Work out the finished part from the listing and answer in its coordinate system (mm). Face numbers are marked on the shaded views. Coordinates: 2 decimals unless noted, no trailing zeros. Write each loop counter-clockwise with the first axis right and the second up, starting at its lowest first coordinate (ties: lowest second). Pieces come first, ordered by that corner, then holes. Notation, with made-up numbers: (85, -3) - (143, -3) arc R11 cw to (143, 17) - close; hole circle Ø5 at (74, 55.25). An arc over 180 degrees is marked (long way). Answer as a JSON object with one key per item and string values. Group by question number.
from build123d import *

# Parameters (mm, degrees)
AUFSATZ_LINEAR_AUSTRAGEN1_DEPTH  = 10
F_3_5_3_5_DURCHMESSER_BOHRUNG2_D = 3.5


with BuildPart() as part:
    # Skizze1 → Aufsatz-Linear austragen1 (new body)
    with BuildSketch(Plane.XY):
        with BuildLine():
            Line((19, 8), (30, 8))
            Line((30, 8), (30, 0))
            Line((30, 0), (0, 0))
            Line((0, 0), (0, 8))
            Line((0, 8), (11, 8))
            ThreePointArc((11, 8), (15, 4), (19, 8))
        make_face()
    extrude(amount=AUFSATZ_LINEAR_AUSTRAGEN1_DEPTH)

    # Ø3.5 (3.5) Durchmesser Bohrung2 (through all)
    with Locations(Plane(origin=(0, 0, 0), x_dir=(-1, 0, 0), z_dir=(0, -1, 0))):
        with Locations((-5, -5), (-25, -5)):
            Hole(F_3_5_3_5_DURCHMESSER_BOHRUNG2_D / 2)


solid = part.part
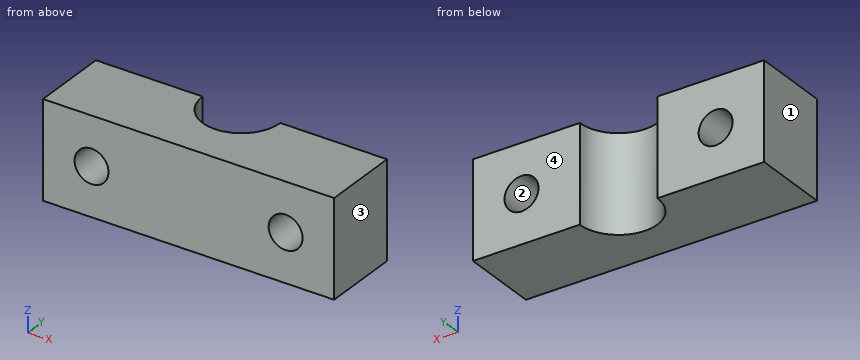
Q1. Section B-B on y = 6.25 is taken. Determine the outline of the cut face in (x, z).
Q2. Section D-D on y = 3.5 is taken. Determine the outline of the cut face in (x, z), plus the area to 3 significant figures.
Q3. Section C-C on x = 5 is taken. Determine the outline of the cut face in (y, z), plus the area to 3 significant figures.
Q4. Section A-A on z = 5 is taken. Determine the outline of the cut face in (x, y).
Q5. Consider L1, parallel to X at y = 2.5, z = 5; L2, parallel to Z at x = 5, y = 2; L3, parallel to X at y = 4.75, z = 5. Determine where each line is inside the solid, lowest interval first. Write a range as from..to.
Q6. For a pull along X with two mould halves and no side action, classify the marked faces 1, 2, 3 and 4 as +X half, -X half, draft (parallel to the pull), parting line (faces both ways), or undercut.
Q7. A flat-ended cylindrical pin translates along its axis: pin 1 Ø6 at (x, z) = (14.5, 3.5) entering from -Y. Find the tip coordinate at first contact, or state that the pin passes through.
Numbers:
{
 "1": {"outline": "(0, 0) - (11.4, 0) - (11.4, 10) - (0, 10) - close; (18.6, 0) - (30, 0) - (30, 10) - (18.6, 10) - close; hole circle Ø3.5 at (5, 5); hole circle Ø3.5 at (25, 5)"},
 "2": {"outline": "(0, 0) - (30, 0) - (30, 10) - (0, 10) - close; hole circle Ø3.5 at (5, 5); hole circle Ø3.5 at (25, 5)", "area": "281 mm²"},
 "3": {"outline": "(0, 0) - (8, 0) - (8, 3.25) - (0, 3.25) - close; (0, 6.75) - (8, 6.75) - (8, 10) - (0, 10) - close", "area": "52.0 mm²"},
 "4": {"outline": "(0, 0) - (3.25, 0) - (3.25, 8) - (0, 8) - close; (6.75, 0) - (23.25, 0) - (23.25, 8) - (19, 8) arc R4 cw to (11, 8) - (6.75, 8) - close; (26.75, 0) - (30, 0) - (30, 8) - (26.75, 8) - close"},
 "5": {"L1": "x = 0..3.25, 6.75..23.25, 26.75..30", "L2": "z = 0..3.25, 6.75..10", "L3": "x = 0..3.25, 6.75..12.67, 17.33..23.25, 26.75..30"},
 "6": {"face 1": "-X half", "face 2": "undercut", "face 3": "+X half", "face 4": "draft"},
 "7": {"pin 1": "stops at y = 0"}
}
